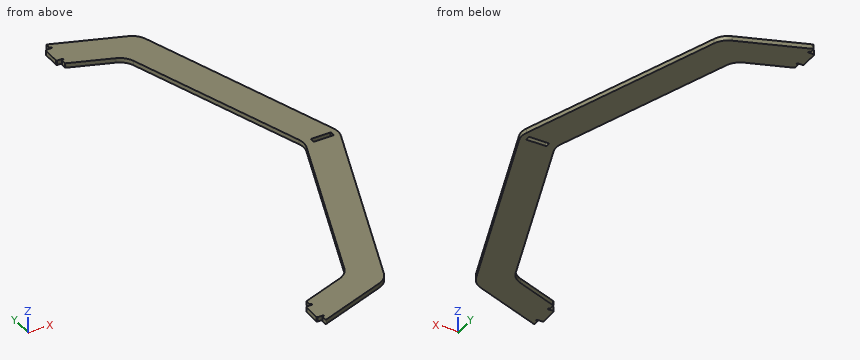
from build123d import *

# Parameters (mm, degrees)
SKETCH1_W           = 13.716
SKETCH1_H           = 3.3528
BOSS_EXTRUDE1_DEPTH = 3.175
FILLET1_R           = 12.7
CUT_EXTRUDE1_DEPTH  = 4.175
FILLET2_R           = 0.508
SCALE1_SCALE        = 0.35


with BuildPart() as part:
    # Sketch1 → Boss-Extrude1 (new body)
    with BuildSketch(Plane.XY):
        Polygon((114.3, 158.75), (114.3, 146.05), (117.475, 146.05), (117.475, 141.224), (151.477068993, 128.848258983), (198.374, 0), (151.477068993, -128.848258983), (117.475, -141.224), (117.475, -146.05), (114.3, -146.05), (114.3, -158.75), (117.475, -158.75), (117.475, -163.576), (169.035670284, -144.809450758), (221.742, 0), (169.035670284, 144.809450758), (117.475, 163.576), (117.475, 158.75), align=None)
        with Locations((210.058, 0)):
            Rectangle(SKETCH1_W, SKETCH1_H, mode=Mode.SUBTRACT)
    extrude(amount=BOSS_EXTRUDE1_DEPTH)

    # Fillet1
    fillet1_edges = [part.edges().sort_by_distance(p)[0] for p in [
        (169.035670284, 144.809450758, 1.5875),
        (221.742, 0, 1.5875),
        (169.035670284, -144.809450758, 1.5875),
        (151.477068993, -128.848258983, 1.5875),
        (198.374, 0, 1.5875),
        (151.477068993, 128.848258983, 1.5875),
    ]]
    fillet(fillet1_edges, radius=FILLET1_R)

    # Sketch2 → Cut-Extrude1 (cut, through all)
    with BuildSketch(Plane.XY.offset(3.175)):
        with BuildLine():
            Line((117.475, 146.05), (118.237, 146.05))
            ThreePointArc((118.237, 146.05), (118.745, 145.542), (118.237, 145.034))
            Line((118.237, 145.034), (117.475, 145.034))
            Line((117.475, 145.034), (117.475, 146.05))
        make_face()
        with BuildLine():
            Line((117.475, 158.75), (118.237, 158.75))
            ThreePointArc((118.237, 158.75), (118.745, 159.258), (118.237, 159.766))
            Line((118.237, 159.766), (117.475, 159.766))
            Line((117.475, 159.766), (117.475, 158.75))
        make_face()
        with BuildLine():
            Line((117.475, -145.034), (117.475, -146.05))
            Line((117.475, -146.05), (118.237, -146.05))
            ThreePointArc((118.237, -146.05), (118.745, -145.542), (118.237, -145.034))
            Line((118.237, -145.034), (117.475, -145.034))
        make_face()
        with BuildLine():
            Line((117.475, -158.75), (117.475, -159.766))
            Line((117.475, -159.766), (118.237, -159.766))
            ThreePointArc((118.237, -159.766), (118.745, -159.258), (118.237, -158.75))
            Line((118.237, -158.75), (117.475, -158.75))
        make_face()
    extrude(amount=-CUT_EXTRUDE1_DEPTH, mode=Mode.SUBTRACT)

    # Fillet2
    fillet2_edges = [part.edges().sort_by_distance(p)[0] for p in [
        (117.475, 163.576, 1.5875),
        (117.475, -163.576, 1.5875),
        (114.3, -158.75, 1.5875),
        (114.3, -146.05, 1.5875),
        (117.475, -141.224, 1.5875),
        (117.475, 141.224, 1.5875),
        (114.3, 146.05, 1.5875),
        (114.3, 158.75, 1.5875),
        (117.475, 159.766, 1.5875),
        (117.475, -159.766, 1.5875),
        (117.475, -145.034, 1.5875),
        (117.475, 145.034, 1.5875),
        (203.2, 1.6764, 1.5875),
        (203.2, -1.6764, 1.5875),
        (216.916, -1.6764, 1.5875),
        (216.916, 1.6764, 1.5875),
    ]]
    fillet(fillet2_edges, radius=FILLET2_R)


with BuildPart() as part_1:
    # Scale1: scaled about (173.96923979, 0, 1.5875)
    add(part.part.scale(SCALE1_SCALE).moved(Location((113.080005863, 0, 1.031875))))


solid = part_1.part
Can you work these out from the model? Positions are in its coordinate system, mm. Give positions to 0.01 mm unless a question says otherwise; leave off trailing zeros. Order: outer loops, then holes, each group sorted by start corner. A loop starts at its lowest first (then second) coordinate and runs counter-clockwise, first axis right, second up. Notation, with made-up numbers: M 42.25,-24.75 L 72.25,-24.75 A21 ccw 72.25,1.25 Z; hole C -30.75,-3.75 d10. An arc over 180 degrees is marked long. Use a Markdown table: item, result. Add a question column.
Item 1: Suppose I cut it at A-A (x = 176). List the corners of the cut face in (y, z) for me, then the cut area to 3 significant figures.
Item 2: Suppose I cut it at B-B (y = -33). List the corners of the cut face in (x, z) for me.
Item 3: Will these pins go through, and if not, where does the flat tip stop? pin 1 (12 mm diameter, centred on x = 164, y = -23.5, fed in from -Z); pin 2 (0.5 mm diameter, centred on y = 50, z = 2, fed in from -X).
Item 4: If I drill on L1, parallel to Y at x = 162, z = 1.95; L2, parallel to Y at x = 165, z = 1.65; L3, parallel to X at y = -39, z = 1.25, over which ranges is the centre line in solid material (lowest first)? Write a range as [from, to].
Answer sheet:
| question | item | result |
|---|---|---|
| 1 | outline | M -40.36,1.03 L -17.89,1.03 L -17.89,2.14 L -40.36,2.14 Z; M 17.89,1.03 L 40.36,1.03 L 40.36,2.14 L 17.89,2.14 Z |
| 1 | area | 49.9 mm² |
| 2 | outline | M 170.5,1.03 L 178.68,1.03 L 178.68,2.14 L 170.5,2.14 Z |
| 3 | pin 1 | passes through |
| 3 | pin 2 | stops at x = 154.2 |
| 4 | L1 | y = [-54.41, -46.59], [46.59, 54.41] |
| 4 | L2 | y = [-53.32, -45.39], [45.39, 53.32] |
| 4 | L3 | x = [168.32, 176.49] |
